Drawing for the job (mm, zero at the part's lowest x, y, z). A direction names the side the tool comes from. Round coordinates to 2 decimals unless told otherwise and drop trailing zeros. Order: outer loops, then holes, each group sorted by start corner. A loop starts at its lowest first (then second) coordinate and runs counter-clockwise, first axis right, second up. Notation, with made-up numbers: (13, 23) - (43, 23) arc R32 ccw to (43, 49) - close; hole circle Ø8 at (82.25, -29.75). An arc over 180 degrees is marked (long way). Put each result on its own line as item: value. Start each with the question number.
Item 1: Pin check, flat tips, straight feed: pin 1 Ø1.5 at (y, z) = (4, 1) entering from +X; pin 2 Ø1.5 at (y, z) = (7.5, 4.5) entering from +X. Stop position of each tip, or through.
Item 2: Saw through at B-B on x = 5. List the corners of the cut face in (y, z) (1 decimal).
Item 3: Saw through at C-C on z = 7. List the corners of the cut face in (x, y) (1 decimal).
Item 4: Saw through at A-A on z = 1.75. List the corners of the cut face in (x, y) (1 decimal).
Item 5: Probe probe 1 along Y at (x, z) = (4.75, 0.5) (1 decimal); probe 2 along X at (y, z) = (3.25, 2.25); probe 3 along X at (y, z) = (3.25, 5.5) (1 decimal). List the from-to ranges inside material, lowest first.
Item 6: Mould opens along Z. For the marked faces 3, 4 and 5 say: pulls with the +Z half, pulls with the -Z half, needs draft (parallel to the pull), parting line crosses it, or undercut.
Item 7: Which spindle directions (+Z, -Z, +X, -X, +Y, -Y) get a long thin tool onto all of the face, cutting with end or side? Do the marked faces 1 and 2. Say none if no direction does.
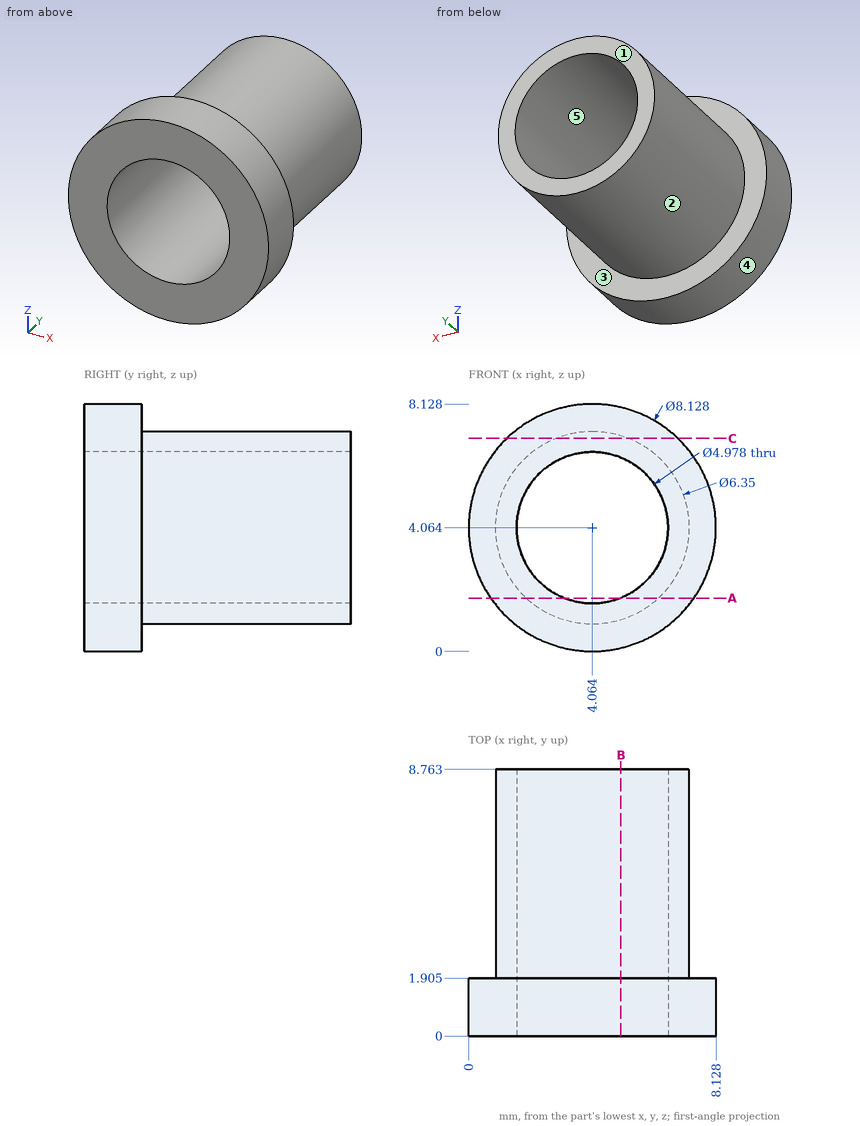
Results found:
1. pin 1: stops at x = 6.24
1. pin 2: stops at x = 7.24
2. outline: (0, 0.1) - (1.9, 0.1) - (1.9, 1) - (8.8, 1) - (8.8, 1.8) - (0, 1.8) - close; (0, 6.4) - (8.8, 6.4) - (8.8, 7.1) - (1.9, 7.1) - (1.9, 8) - (0, 8) - close
3. outline: (1.3, 0) - (6.9, 0) - (6.9, 1.9) - (5.3, 1.9) - (5.3, 8.8) - (2.9, 8.8) - (2.9, 1.9) - (1.3, 1.9) - close
4. outline: (0.7, 0) - (3.1, 0) - (3.1, 8.8) - (1.9, 8.8) - (1.9, 1.9) - (0.7, 1.9) - close; (5, 0) - (7.4, 0) - (7.4, 1.9) - (6.2, 1.9) - (6.2, 8.8) - (5, 8.8) - close
5. probe 1: y = 0 to 1.9
5. probe 2: x = 1.46 to 2.36, 5.77 to 6.67
5. probe 3: x = 1.2 to 2, 6.1 to 6.9
6. face 3: needs draft
6. face 4: parting line crosses it
6. face 5: undercut
7. face 1: +Z, -Z, +X, -X, +Y
7. face 2: +Y
